```python
from build123d import *

# Parameters (mm, degrees)
F1_ANGLE_BACK = 90
F1_ANGLE      = 180
F2_T          = 1
F2_T4_ANGLE   = 180.000000001
F2_T6_ANGLE   = 180.000000001
F3_R          = 1
F4_R          = 0.5


# Not quite as in the source:
# - a feature of the source that left no trace in its solid (it failed there, or was rolled back) is left out
# - a shell that OpenCascade refuses in one call is made with other operations: the cavity is built on its own and cut out


with BuildPart() as f1:
    # F0 (on Top) → F1 (revolve)
    with BuildSketch(Plane.XY, mode=Mode.PRIVATE) as f1_sk:
        Polygon((-2.5, 1.5875), (-5, 1.5875), (-5, 0), (5, 0), (5, 1.5875), (2.5, 1.5875), (2.5, 3), (-2.5, 3), align=None)
    revolve(f1_sk.sketch.rotate(Axis((0.2477309544, 0, 0), (1, 0, 0)), -F1_ANGLE_BACK), axis=Axis((0.2477309544, 0, 0), (1, 0, 0)), revolution_arc=F1_ANGLE)

    # F2: shell of thickness 1, made by hand


with BuildPart() as f2_core1:
    # F2_t2: copy of F1
    add(f1.part)

    # the walls: a layer under each face that stays
    f2_faces = [f2_core1.faces().sort_by_distance(p)[0] for p in [
        (-3.75, 1.5875, 0),
        (0, 0, 0),
        (3.75, 1.5875, 0),
        (2.5, 0.5, -2),
        (0, 3, 0),
        (-2.5, 0.5, 2),
    ]]
    thicken(f2_faces, amount=-F2_T, mode=Mode.SUBTRACT)

    # F2_s3 → F2_t4 (revolve, cut)
    with BuildSketch(Plane.XZ):
        Polygon((-2.51, -1.5975), (-2.5, -0.5875), (-1.5, -0.5875), (-1.5, -1.5875), align=None)
    revolve(axis=Axis((-2.5, 0, 0), (1, 0, 0)), revolution_arc=F2_T4_ANGLE, mode=Mode.SUBTRACT)

    # F2_s5 → F2_t6 (revolve, cut)
    with BuildSketch(Plane.XZ):
        Polygon((2.51, -1.5975), (2.5, -0.5875), (1.5, -0.5875), (1.5, -1.5875), align=None)
    revolve(axis=Axis((2.5, 0, 0), (1, 0, 0)), revolution_arc=F2_T6_ANGLE, mode=Mode.SUBTRACT)


with BuildPart() as f1_1:
    add(f1.part)

    # what is left inside the walls is the cavity
    f2_cavity = [f2_core1.part.solids().sort_by_distance(p)[0] for p in [
        (0.5, 1.99, 0),
    ]]
    add(f2_cavity, mode=Mode.SUBTRACT)

    # F3
    f3_edges = [f1_1.edges().sort_by_distance(p)[0] for p in [
        (5, 1.5875, 0),
    ]]
    fillet(f3_edges, radius=F3_R)

    # F4
    f4_edges = [f1_1.edges().sort_by_distance(p)[0] for p in [
        (-5, 1.5875, 0),
    ]]
    fillet(f4_edges, radius=F4_R)


solid = f1_1.part
```
Read the model definition and answer for the solid it produces. Units are mm, in the model's axes. A direction names the side the tool comes from. Coordinates: 2 decimals unless noted, no trailing zeros. Write each loop counter-clockwise with the first axis right and the second up, starting at its lowest first coordinate (ties: lowest second). Pieces come first, ordered by that corner, then holes. Notation, with made-up numbers: (20.25, 72) -> (37.25, 72) arc R25 cw to (37.25, 97) -> close; hole circle Ø2 at (57.5, 79). An arc over 180 degrees is marked (long way). Answer as a JSON object with one key per item and string values.
Q1. Flat-ended cylindrical pins translate along their axes: pin 1 Ø0.5 at (y, z) = (1.5, -0.5) entering from -X; pin 2 Ø0.9 at (y, z) = (2, -1) entering from +X; pin 3 Ø0.5 at (y, z) = (1.5, 0.5) entering from +X. Find the tip coordinate at first contact, or state that the pin passes through.
The answers:
{"pin 1": "stops at x = -4.94", "pin 2": "stops at x = 2.5", "pin 3": "stops at x = 4.67"}
Q2. A tool of negligible diameter and unlimited length cuts with its end or side. For faces 5 (the flat face through (-1.5, 1.4, 0)), 6 (the cylindrical face through (-3.514, 1.587, -0.035)), 7 (the cylindrical face through (3.24, 1.587, -0.035)), from which of +Z, -Z, +X, -X, +Y, -Y can it reach the whole face along a straight path? Write none if from no direction.
The answers:
{"face 5": "none", "face 6": "-X, +Y", "face 7": "+X, +Y"}
Q3. The part is cut by section D-D on z = -2. Give the vertices of the cut face in (x, y).
The answers:
{"outline": "(-2.5, 0) -> (2.5, 0) -> (2.5, 2.24) -> (-2.5, 2.24) -> close"}
Q4. The part is cut by section B-B on x = 2.75. Give the vertices of the cut face in (y, z) (1 decimal).
The answers:
{"outline": "(0, -1.6) arc R1.6 ccw to (0, 1.6) -> close"}
Q5. Consider line 1 (X direction, y = 1.85, z = 0.5); line 2 (X direction, y = 1.25, z = 2.5); line 3 (Y direction, x = 0.5, z = -1). Determine where each line is inside the solid, lowest interval first. Write a range as [from, to].
The answers:
{"line 1": "x = [-2.5, -1.5], [1.5, 2.5]", "line 2": "x = [-2.5, 2.5]", "line 3": "y = [0, 1], [1.73, 2.83]"}
Q6. The part is cut by section A-A on y = 1.7. Give the vertices of the cut face in (x, z), then the cut area to 3 significant figures.
The answers:
{"outline": "(-2.5, -2.47) -> (2.5, -2.47) -> (2.5, 2.47) -> (-2.5, 2.47) -> close; hole (-1.5, -1.05) -> (1.5, -1.05) -> (1.5, 1.05) -> (-1.5, 1.05) -> close", "area": "18.4 mm2"}
Q7. Determine the mould class of faces 1 (the flat face through (0, 0, 0)), 2 (the flat face through (-2.5, 2, 0)), 3 (the flat face through (0, 1, 0)), 4 (the flat face through (1.5, 1.4, 0)) for opening direction X: pulls with the +X half, pulls with the -X half, needs draft (parallel to the pull), parting line crosses it, or undercut.
The answers:
{"face 1": "needs draft", "face 2": "pulls with the -X half", "face 3": "undercut", "face 4": "undercut"}
Q8. The part is cut by section C-C on x = -0.5. Give the vertices of the cut face in (y, z), then the cut area to 3 significant figures.
The answers:
{"outline": "(0, -3) arc R3 ccw to (0, 3) -> close; hole (1, -1.73) arc R2 ccw to (1, 1.73) -> close", "area": "11.7 mm2"}
